from build123d import *

# Parameters (mm, degrees)
SKETCH1_R           = 15
SKETCH1_R_2         = 1
BOSS_EXTRUDE1_DEPTH = 4
CUT_EXTRUDE1_DEPTH  = 0.5


with BuildPart() as part:
    # Sketch1 → Boss-Extrude1 (new, symmetric)
    with BuildSketch(Plane.XY):
        Circle(SKETCH1_R)
        Circle(SKETCH1_R_2, mode=Mode.SUBTRACT)
    extrude(amount=BOSS_EXTRUDE1_DEPTH, both=True)

    # Sketch2 → Cut-Extrude1 (cut)
    with BuildSketch(Plane.XY.offset(4)):
        Polygon((-4.330127019, 7.5), (-8.660254038, 0), (-4.330127019, -7.5), (4.330127019, -7.5), (8.660254038, 0), (4.330127019, 7.5), align=None)
    extrude(amount=-CUT_EXTRUDE1_DEPTH, mode=Mode.SUBTRACT)


solid = part.part
Geometry: final body of the model. Coordinates: model frame, mm. A direction names the side the tool comes from. Coordinates: 2 decimals unless noted, no trailing zeros. Order: outer loops, then holes, each group sorted by start corner. A loop starts at its lowest first (then second) coordinate and runs counter-clockwise, first axis right, second up.
(1) Section query A-A (x = 0). Return the cut outline in (y, z).
(2) Section query B-B (y = -2.5). Return the cut outline in (x, z).
(3) Section query C-C (z = -2.75). Return the cut outline in (x, y).
(4) First-contact query: pin 1 (3 mm diameter, centred on x = 0, y = 0, fed in from -Z); pin 2 (3 mm diameter, centred on x = -3, z = 2, fed in from -Y); pin 3 (4 mm diameter, centred on y = -7, z = -2, fed in from +X); pin 4 (7.5 mm diameter, centred on x = -1, y = -2, fed in from +Z). Flat tips, straight axial feed; report the tip coordinate or a pass-through.
(5) Access query for faces 1 (the face through (-6.526, -3.698, 3.754)), 2 (the face through (3, 0, -4)). Directions: +Z, -Z, +X, -X, +Y, -Y. A direction counts if a zero-diameter tool reaches every point of the face in a straight line with its end or side. Return the directions, or none.
(6) Section query D-D (y = 3). Return the cut outline in (x, z), plus the area to 3 significant figures.
(7) Material intervals for probe 1 along Y at (x, z) = (0, 0); probe 2 along Z at (x, y) = (-0.75, 2.25); probe 3 along Y at (x, z) = (4, -2.25), sorted ascending.
(8) Draft query along X for faces 3 (the face through (-7, 4, 4)), 4 (the face through (-14.985, 0.66, 0.056)), 5 (the face through (6.526, 3.698, 3.754)). Return one class per face: pulls with the +X half, pulls with the -X half, needs draft (parallel to the pull), parting line crosses it, or undercut.
Solution:
1. outline: (-15, -4) - (-1, -4) - (-1, 3.5) - (-7.5, 3.5) - (-7.5, 4) - (-15, 4) - close; (1, -4) - (15, -4) - (15, 4) - (7.5, 4) - (7.5, 3.5) - (1, 3.5) - close
2. outline: (-14.79, -4) - (14.79, -4) - (14.79, 4) - (7.22, 4) - (7.22, 3.5) - (-7.22, 3.5) - (-7.22, 4) - (-14.79, 4) - close
3. outline: circle Ø30 at (0, 0); hole circle Ø2 at (0, 0)
4. pin 1: stops at z = -4
4. pin 2: stops at y = -14.92
4. pin 3: stops at x = 14.14
4. pin 4: stops at z = 3.5
5. face 1: +Z
5. face 2: -Z, +X, -X, +Y, -Y
6. outline: (-14.7, -4) - (14.7, -4) - (14.7, 4) - (6.93, 4) - (6.93, 3.5) - (-6.93, 3.5) - (-6.93, 4) - (-14.7, 4) - close
6. area: 228 mm2
7. probe 1: y = -15 to -1, 1 to 15
7. probe 2: z = -4 to 3.5
7. probe 3: y = -14.46 to 14.46
8. face 3: needs draft
8. face 4: parting line crosses it
8. face 5: undercut
